from build123d import *

# Parameters (mm, degrees)
F0_W     = 11
F0_H     = 25
F1_DEPTH = 7
F3_DEPTH = 11
F4_R     = 1.8
F5_DEPTH = 7
F6_SIZE  = 0.5


with BuildPart() as f1:
    # F0 (on Top) → F1 (new body)
    with BuildSketch(Plane.XY):
        Rectangle(F0_W, F0_H)
    extrude(amount=F1_DEPTH)

    # F2 (on face) → F3 (cut, through all)
    with BuildSketch(Plane.YZ.offset(5.5)):
        with BuildLine():
            Line((-4.1892720131, 0), (4.1892720131, 0))
            ThreePointArc((4.1892720131, 0), (0, 3.9), (-4.1892720131, 0))
        make_face()
    extrude(amount=-F3_DEPTH, mode=Mode.SUBTRACT)

    # F4 (on face) → F5 (cut, through all)
    with BuildSketch(Plane(origin=(0, 0, 0), x_dir=(1, 0, 0), z_dir=(0, 0, -1))):
        with Locations((0, 8.3446360066)):
            Circle(F4_R)
        with Locations((0, -8.3446360066)):
            Circle(F4_R)
    extrude(amount=-F5_DEPTH, mode=Mode.SUBTRACT)

    # F6
    f6_edges = [f1.edges().sort_by_distance(p)[0] for p in [
        (5.5, 0, 3.9),
        (5.5, 8.344636, 0),
        (0, 12.5, 0),
        (-5.5, 8.344636, 0),
        (5.5, -8.344636, 0),
        (0, -12.5, 0),
        (-5.5, -8.344636, 0),
        (5.5, -12.5, 3.5),
        (0, -12.5, 7),
        (-5.5, -12.5, 3.5),
        (5.5, 0, 7),
        (5.5, 12.5, 3.5),
        (0, 12.5, 7),
        (-5.5, 12.5, 3.5),
        (-5.5, 0, 7),
        (-5.5, 0, 3.9),
    ]]
    chamfer(f6_edges, length=F6_SIZE)


solid = f1.part
The model under review builds one solid part; all positions refer to its coordinate system, in mm. Coordinates: 2 decimals unless noted, no trailing zeros. Loops run counter-clockwise (first coordinate to the right, second up) from the corner with the lowest first, then second, coordinate; pieces in that order, holes last. Notation, with made-up numbers: M 67,79.25 L 101,79.25 A27 ccw 101,111.25 Z; hole C 6.5,78.25 d5. An arc over 180 degrees is marked long. Put each result on its own line as item: value. Start each with the question number.
Q1. Clearance check with flat-ended pins moving along their axes: pin 1 (3 mm diameter, centred on x = 0, y = 8.34, fed in from +Z); pin 2 (3 mm diameter, centred on x = 2, y = 1.5, fed in from -Z). State where each tip first meets the part, or that it passes through.
Q2. Add section C-C (x = 4). Write out the cut boundary in (y, z), and give its area (3 significant figures).
Q3. Add section D-D (z = 5.5). Write out the cut boundary in (x, y), and give its area (3 significant figures).
Q4. Add section A-A (x = 0). Write out the cut boundary in (y, z).
Q5. The part is to be moulded in two halves that separate along Y. For faces 1 (the flat face through (-5.5, 0, 5)), 2 (the cylindrical face through (-0.23, 6.56, 3.45)), 3 (the flat face through (0, -12.5, 3)), 4 (the flat face through (0, 12.5, 3)), say which applies: +Y half, -Y half, draft (parallel to the pull), parting line (faces both ways), or undercut.
Q6. Wall thickness on line 1 (Y direction, x = 0, z = 4.5); line 2 (Y direction, x = 0, z = 1.5); line 3 (Y direction, x = 0, z = 3.5): over which ranges is each line inside the solid? List them lowest first.
Q7. Add section B-B (y = 9.5). Write out the cut boundary in (x, z), and give its area (3 significant figures).
Answers:
1. pin 1: passes through
1. pin 2: stops at z = 2.64
2. outline: M -12.5,0.5 L -12,0 L -4.19,0 A4.2 cw 4.19,0 L 12,0 L 12.5,0.5 L 12.5,6.5 L 12,7 L -12,7 L -12.5,6.5 Z
2. area: 149 mm^2
3. outline: M -5.5,-12 L -5,-12.5 L 5,-12.5 L 5.5,-12 L 5.5,12 L 5,12.5 L -5,12.5 L -5.5,12 Z; hole C 0,-8.34 d3.6; hole C 0,8.34 d3.6
3. area: 254 mm^2
4. outline: M -12.5,0.5 L -12,0 L -10.14,0 L -10.14,7 L -12,7 L -12.5,6.5 Z; M -6.54,0 L -4.19,0 A4.2 cw 4.19,0 L 6.54,0 L 6.54,7 L -6.54,7 Z; M 10.14,0 L 12,0 L 12.5,0.5 L 12.5,6.5 L 12,7 L 10.14,7 Z
5. face 1: draft
5. face 2: undercut
5. face 3: -Y half
5. face 4: +Y half
6. line 1: y = -12.5 to -10.14, -6.54 to 6.54, 10.14 to 12.5
6. line 2: y = -12.5 to -10.14, -6.54 to -3.79, 3.79 to 6.54, 10.14 to 12.5
6. line 3: y = -12.5 to -10.14, -6.54 to -1.79, 1.79 to 6.54, 10.14 to 12.5
7. outline: M -5.5,0.5 L -5,0 L -1.38,0 L -1.38,7 L -5,7 L -5.5,6.5 Z; M 1.38,0 L 5,0 L 5.5,0.5 L 5.5,6.5 L 5,7 L 1.38,7 Z
7. area: 57.2 mm^2
